Input: part model. Units: mm. Frame: model coordinates. Face numbers are marked on the shaded views. A direction names the side the tool comes from. Coordinates: 2 decimals unless noted, no trailing zeros. Order: outer loops, then holes, each group sorted by start corner. A loop starts at its lowest first (then second) coordinate and runs counter-clockwise, first axis right, second up. Notation, with made-up numbers: (23.25, 20) -> (81.25, 20) arc R24 cw to (81.25, 38) -> close; hole circle Ø2 at (87.5, 76). An arc over 180 degrees is marked (long way). One line per question, with ' | ' between items.
```python
from build123d import *

# Parameters (mm, degrees)
F1_DEPTH  = 25
F2_W      = 8
F2_H      = 18
F3_DEPTH  = 25.001
F4_W      = 35
F4_H      = 16
F5_DEPTH  = 246.8787132738
F7_DEPTH  = 25
F8_SIZE   = 1
F9_SIZE   = 1
F10_SIZE  = 1
F11_SIZE  = 1
F12_SIZE  = 1
F13_R     = 10
F14_DEPTH = 25.001


with BuildPart() as f1:
    # F0 (on Top) → F1 (new body)
    with BuildSketch(Plane.XY):
        Polygon((-392, 0), (0, 0), (0, 246.8777132738), (-80, 246.8777132738), (-80, 130), (-392, 130), align=None)
    extrude(amount=F1_DEPTH)

    # F2 (on face) → F3 (cut, through all)
    with BuildSketch(Plane.XY.offset(25)):
        with Locations((-388, 106)):
            Rectangle(F2_W, F2_H)
        with Locations((-388, 55)):
            Rectangle(F2_W, F2_H)
    extrude(amount=-F3_DEPTH, mode=Mode.SUBTRACT)

    # F4 (on face) → F5 (cut, through all)
    with BuildSketch(Plane.XZ):
        with Locations((-374.5, 8)):
            Rectangle(F4_W, F4_H)
    extrude(amount=-F5_DEPTH, mode=Mode.SUBTRACT)

    # F6 (on face) → F7 (join)
    with BuildSketch(Plane.XY.offset(25)):
        Polygon((-355.1386892796, 10), (-355.1386892796, 0), (0, 0), (0, 246.8777132738), (-10, 246.8777132738), (-10, 10), align=None)
    extrude(amount=F7_DEPTH)

    # F8
    f8_edges = [f1.edges().sort_by_distance(p)[0] for p in [
        (-392, 23, 25),
        (-384, 55, 25),
        (-392, 80.5, 25),
        (-384, 106, 25),
        (-392, 122.5, 25),
        (-388, 64, 25),
        (-388, 46, 25),
        (-388, 115, 25),
        (-388, 97, 25),
    ]]
    chamfer(f8_edges, length=F8_SIZE)

    # F9
    f9_edges = [f1.edges().sort_by_distance(p)[0] for p in [
        (-235.5, 130, 25),
        (-80, 188.438857, 25),
    ]]
    chamfer(f9_edges, length=F9_SIZE)

    # F10
    f10_edges = [f1.edges().sort_by_distance(p)[0] for p in [
        (-182.569345, 10, 50),
        (-10, 128.438857, 50),
    ]]
    chamfer(f10_edges, length=F10_SIZE)

    # F11
    f11_edges = [f1.edges().sort_by_distance(p)[0] for p in [
        (-355.138689, 10, 37),
    ]]
    chamfer(f11_edges, length=F11_SIZE)

    # F12
    f12_edges = [f1.edges().sort_by_distance(p)[0] for p in [
        (-44.5, 246.877713, 25),
        (-10, 246.877713, 37),
    ]]
    chamfer(f12_edges, length=F12_SIZE)

    # F13 (on face) → F14 (cut, through all)
    with BuildSketch(Plane.XY.offset(25)):
        with BuildLine():
            ThreePointArc((-46.8990951777, 63.3794814348), (-56.8990951777, 73.3794814348), (-66.8990951777, 63.3794814348))
            ThreePointArc((-66.8990951777, 63.3794814348), (-56.8990951777, 53.3794814348), (-46.8990951777, 63.3794814348))
        make_face()
        with Locations((-171.8990951777, 63.3794814348)):
            Circle(F13_R)
    extrude(amount=-F14_DEPTH, mode=Mode.SUBTRACT)


solid = f1.part
```
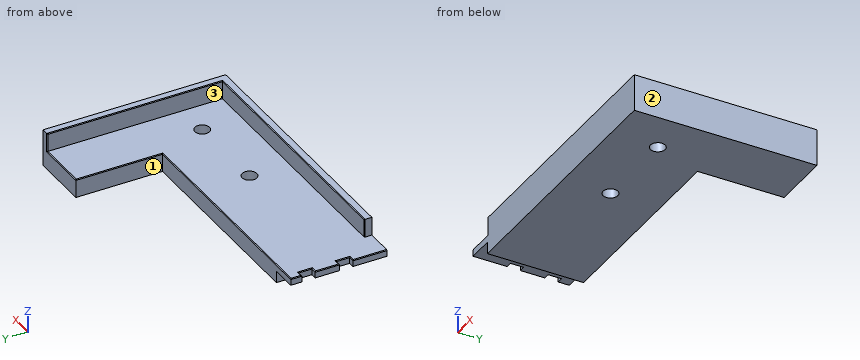
1. Cut plane C-C, the plane z = 45. Return loops of the section in (x, y).
Recorded:
outline: (-355.14, 0) -> (0, 0) -> (0, 246.88) -> (-9, 246.88) -> (-10, 245.88) -> (-10, 10) -> (-354.14, 10) -> (-355.14, 9) -> close
2. Cut plane D-D, the plane z = 5. Return loops of the section in (x, y).
Recorded:
outline: (-357, 0) -> (0, 0) -> (0, 246.88) -> (-80, 246.88) -> (-80, 130) -> (-357, 130) -> close; hole circle Ø20 at (-171.9, 63.38); hole circle Ø20 at (-56.9, 63.38)
3. Cut plane A-A, the plane y = 27.5. Return loops of the section in (x, z), and give its area (3 significant figures).
Recorded:
outline: (-392, 16) -> (-357, 16) -> (-357, 0) -> (0, 0) -> (0, 50) -> (-9, 50) -> (-10, 49) -> (-10, 25) -> (-391, 25) -> (-392, 24) -> close | area: 9,490 mm^2
4. Access query for the marked faces 1, 2 and 3. Directions: +Z, -Z, +X, -X, +Y, -Y. A direction counts if a zero-diameter tool reaches every point of the face in a straight line with its end or side. Return the directions, or none.
Recorded:
face 1: +Z, -Z, -X, +Y | face 2: +Z, -Z, +X, +Y, -Y | face 3: +Z, -X, +Y
5. Pin query (flat end, axial travel): pin 1 Ø4 at (x, z) = (-388.5, 21) entering from +Y; pin 2 Ø1 at (x, z) = (-314.5, 38) entering from +Y; pin 3 Ø2.5 at (y, z) = (58.5, 19) entering from -X. Return the tip coordinate at first contact, or that it passes through.
Recorded:
pin 1: stops at y = 130 | pin 2: stops at y = 10 | pin 3: stops at x = -384
6. Ray query, line 1 (Y direction, x = -230, z = 44); line 2 (X direction, y = 29, z = 10); line 3 (Z direction, x = -267, y = 42.5). Return the intervals inside material, ascending. Write a range as [from, to].
Recorded:
line 1: y = [0, 10] | line 2: x = [-357, 0] | line 3: z = [0, 25]
7. Cut plane B-B, the plane x = -109.5. Return loops of the section in (y, z).
Recorded:
outline: (0, 0) -> (130, 0) -> (130, 24) -> (129, 25) -> (10, 25) -> (10, 49) -> (9, 50) -> (0, 50) -> close
